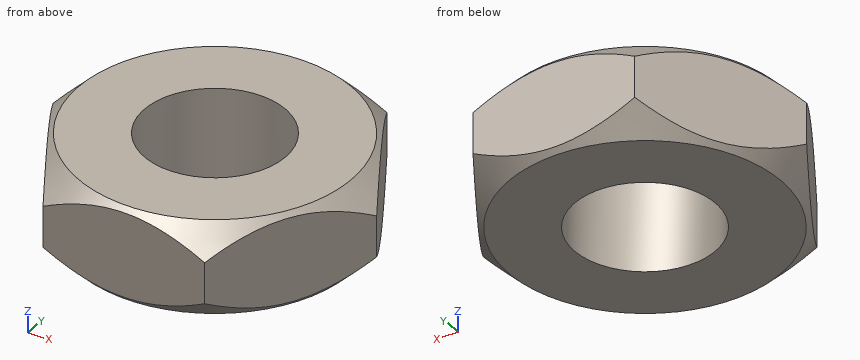
```python
from build123d import *

# Parameters (mm, degrees)
SKETCH_R  = 1.5
PAD_DEPTH = 1


with BuildPart() as part:
    # Sketch → Pad (new body, symmetric)
    with BuildSketch(Plane.XY):
        Polygon((3.464102, 0), (1.732051, 3), (-1.732051, 3), (-3.464102, 0), (-1.732051, -3), (1.732051, -3), align=None)
        Circle(SKETCH_R, mode=Mode.SUBTRACT)
    extrude(amount=PAD_DEPTH, both=True)

    # Sketch001 → Groove (revolve, cut)
    with BuildSketch(Plane.YZ):
        Polygon((2.05363, 1.852295), (2.05363, 2.729858), (5.279402, 2.729858), (5.279402, -3.14441), (2.05363, -3.14441), (2.05363, -1.840465), (3.9, 0), align=None)
    revolve(axis=Axis((0, 0, 0), (0, 0, 1)), mode=Mode.SUBTRACT)


solid = part.part
```
Geometry check sheet. Reference: the model listing, model coordinates, mm. Round coordinates to 2 decimals unless told otherwise and drop trailing zeros. Loops run counter-clockwise (first coordinate to the right, second up) from the corner with the lowest first, then second, coordinate; pieces in that order, holes last. Notation, with made-up numbers: M 20,80.5 L 62,80.5 A16 ccw 62,94.5 Z; hole C 52.25,17.25 d3. An arc over 180 degrees is marked long. Return JSON: item names as keys, results as strings. Group by question number.
(1) Section check A-A, the plane x = 0. Enter the section's corners in (y, z).
(2) Scan lines: line 1 along Y through (x, z) = (0, 0.1); line 2 along Y through (x, z) = (1.25, -0.7); line 3 along X through (y, z) = (-0.25, 0.6). Record each from-to range of solid material in increasing order. Write a range as [from, to].
(3) Section check B-B, the plane z = -0.35. Enter the section's corners in (x, y), and give its area (3 significant figures).
Data:
{
 "1": {"outline": "M -3,-0.9 L -2.9,-1 L -1.5,-1 L -1.5,1 L -2.9,1 L -3,0.9 Z; M 1.5,-1 L 2.9,-1 L 3,-0.9 L 3,0.9 L 2.9,1 L 1.5,1 Z"},
 "2": {"line 1": "[-3, -1.5], [1.5, 3]", "line 2": "[-2.94, -0.83], [0.83, 2.94]", "line 3": "[-3.29, -1.48], [1.48, 3.29]"},
 "3": {"outline": "M -3.46,0 L -1.73,-3 L 1.73,-3 L 3.46,0 L 1.73,3 L -1.73,3 Z; hole C 0,0 d3", "area": "24.1 mm²"}
}
